```python
from build123d import *

# Parameters (mm, degrees)
F0_R     = 22.225
F1_DEPTH = 76.2
F4_D     = 34.29
F4_DEPTH = 50.801
F6_D     = 25.4


with BuildPart() as f1:
    # F0 (on Front) → F1 (new body)
    with BuildSketch(Plane.XZ):
        with BuildLine():
            Line((-149.225, 0), (0, 0))
            Line((0, 0), (0, 50.8))
            Line((0, 50.8), (-76.2, 50.8))
            Line((-76.2, 50.8), (-76.2, 101.6))
            Line((-76.2, 101.6), (0, 101.6))
            Line((0, 101.6), (0, 152.4))
            Line((0, 152.4), (-149.225, 152.4))
            ThreePointArc((-149.225, 152.4), (-225.425, 76.2), (-149.225, 0))
        make_face()
        with Locations((-114.3, 76.2)):
            Circle(F0_R, mode=Mode.SUBTRACT)
    extrude(amount=F1_DEPTH)

    # F4 (through all, one way)
    with BuildSketch(Plane.XY.offset(50.8)):
        with Locations((-38.1, -38.1)):
            Circle(F4_D / 2)
    extrude(amount=-F4_DEPTH, mode=Mode.SUBTRACT)

    # F6 (through all)
    with Locations(Plane.XY.offset(152.4)):
        with Locations((-38.1, -38.1)):
            Hole(F6_D / 2)


solid = f1.part
```
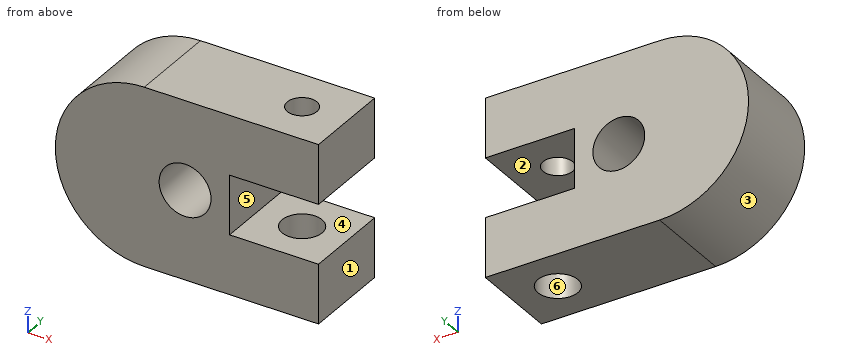
Geometry check sheet. Reference: the model listing, model coordinates, mm. Face numbers are marked on the shaded views. A direction names the side the tool comes from. Coordinates: 2 decimals unless noted, no trailing zeros. Loops run counter-clockwise (first coordinate to the right, second up) from the corner with the lowest first, then second, coordinate; pieces in that order, holes last. Notation, with made-up numbers: (40.5, 19) - (79.5, 19) arc R14 cw to (79.5, 23) - close; hole circle Ø1 at (27, 51). An arc over 180 degrees is marked (long way). One line per item, written item: value. Start each with the question number.
(1) Depth check by flat-ended pin: P1, Ø2, axis at y = -45.5, z = 84.5, coming from the -X side; P2, Ø5, axis at x = -178.5, y = -59, coming from the +Z side. Enter the tip coordinate at first touch or a pass-through.
(2) Cross-section at D-D on x = -114.3. Enter the section's corners in (y, z) (3 decimals), plus the area to 3 significant figures.
(3) Cross-section at B-B on y = -38.1. Enter the section's corners in (x, z) (3 decimals).
(4) Cross-section at C-C on z = 76.2. Enter the section's corners in (x, y) (3 decimals), plus the area to 3 significant figures.
(5) Cross-section at A-A on x = -38.1. Enter the section's corners in (y, z) (3 decimals), plus the area to 3 significant figures.
(6) Material ranges on line 1 (Z direction, x = -114, y = -18); line 2 (Z direction, x = -58.5, y = -10.5); line 3 (X direction, y = -61.5, z = 90.5), recorded low to high. Write a range as [from, to].
(7) Tool access check on the marked faces 1 and 2. Record the directions out of +Z, -Z, +X, -X, +Y, -Y that give a thin tool (end or side, any length) a straight path to the whole face; none if there is none.
(8) Mould release check, pull along X, two halves, no side actions. Record for the marked faces 3, 4, 5 and 6: released by +X, released by -X, zero draft, split by the parting line, or undercut.
Results below:
1. P1: stops at x = -225.07
1. P2: stops at z = 147.54
2. outline: (-76.2, 0) - (0, 0) - (0, 53.975) - (-76.2, 53.975) - close; (-76.2, 98.425) - (0, 98.425) - (0, 152.4) - (-76.2, 152.4) - close
2. area: 8,230 mm2
3. outline: (-149.225, 0) - (-55.245, 0) - (-55.245, 50.8) - (-76.2, 50.8) - (-76.2, 101.6) - (-50.8, 101.6) - (-50.8, 152.4) - (-149.225, 152.4) arc R76.2 ccw to start; (-25.4, 101.6) - (0, 101.6) - (0, 152.4) - (-25.4, 152.4) - close; (-20.955, 0) - (0, 0) - (0, 50.8) - (-20.955, 50.8) - close; hole circle Ø44.45 at (-114.3, 76.2)
4. outline: (-225.425, -76.2) - (-136.525, -76.2) - (-136.525, 0) - (-225.425, 0) - close; (-92.075, -76.2) - (-76.2, -76.2) - (-76.2, 0) - (-92.075, 0) - close
4. area: 7,980 mm2
5. outline: (-76.2, 0) - (-55.245, 0) - (-55.245, 50.8) - (-76.2, 50.8) - close; (-76.2, 101.6) - (-50.8, 101.6) - (-50.8, 152.4) - (-76.2, 152.4) - close; (-25.4, 101.6) - (0, 101.6) - (0, 152.4) - (-25.4, 152.4) - close; (-20.955, 0) - (0, 0) - (0, 50.8) - (-20.955, 50.8) - close
5. area: 4,710 mm2
6. line 1: z = [0, 53.98], [98.42, 152.4]
6. line 2: z = [0, 50.8], [101.6, 152.4]
6. line 3: x = [-224.07, -131.31], [-97.29, -76.2]
7. face 1: +Z, -Z, +X, +Y, -Y
7. face 2: +X, +Y, -Y
8. face 3: released by -X
8. face 4: zero draft
8. face 5: released by +X
8. face 6: undercut
